```python
from build123d import *

# Parameters (mm, degrees)
SKETCH_1_W          = 25
SKETCH_1_H          = 2
EXTRUDE_1_DEPTH     = 20
SKETCH_1_3_W        = 25
SKETCH_1_3_H        = 10
SKETCH_1_3_R        = 1.5
EXTRUDE_2_DEPTH     = 2
SKETCH_2_R          = 1.5
CUT_EXTRUDE_1_DEPTH = 2


with BuildPart() as part:
    # Sketch 1 → Extrude 1 (new body)
    with BuildSketch(Plane(origin=(0, 0, 0), x_dir=(1, 0, 0), z_dir=(0, 1, 0))):
        with Locations((0, 4)):
            Rectangle(SKETCH_1_W, SKETCH_1_H)
    extrude(amount=EXTRUDE_1_DEPTH)

    # Sketch 1_3 → Extrude 2 (add)
    with BuildSketch(Plane(origin=(0, 0, 0), x_dir=(1, 0, 0), z_dir=(0, 1, 0))):
        Rectangle(SKETCH_1_3_W, SKETCH_1_3_H)
        with Locations(Location((-7.5, 0.997487313, 0), (0, 0, 270))):
            Circle(SKETCH_1_3_R, mode=Mode.SUBTRACT)
        with Locations(Location((7.5, 0.997487313, 0), (0, 0, 270))):
            Circle(SKETCH_1_3_R, mode=Mode.SUBTRACT)
    extrude(amount=EXTRUDE_2_DEPTH)

    # Sketch 2 → Cut-Extrude 1 (cut)
    with BuildSketch(Plane.XY.offset(-3)):
        with Locations((-7.5, 16.745611825)):
            Circle(SKETCH_2_R)
        with Locations((7.5, 16.745611825)):
            Circle(SKETCH_2_R)
    extrude(amount=-CUT_EXTRUDE_1_DEPTH, mode=Mode.SUBTRACT)


solid = part.part
```
CAD build for the part. Positions are in the model's coordinates, mm. A direction names the side the tool comes from. Coordinates: 2 decimals unless noted, no trailing zeros. Order: outer loops, then holes, each group sorted by start corner. A loop starts at its lowest first (then second) coordinate and runs counter-clockwise, first axis right, second up. Notation, with made-up numbers: (84.25, 16) - (111.25, 16) arc R32 cw to (111.25, 44) - close; hole circle Ø11 at (72.25, 8). An arc over 180 degrees is marked (long way). Use a Markdown table: item, result. Add a question column.
(1) Pull direction Z, two halves, no side cores. Call faces 1 (the face through (0, 0, 0)), 2 (the face through (0, 11, -3)), 3 (the face through (-9, 1, -1)): +Z half, -Z half, draft (parallel to the pull), parting line (faces both ways), or undercut.
(2) Flat gauge pins, fed straight in: pin 1 (3 mm diameter, centred on x = -8.5, y = 17, fed in from -Z); pin 2 (2.5 mm diameter, centred on x = -2, z = 0.5, fed in from +Y); pin 3 (1 mm diameter, centred on x = 0, y = 3.5, fed in from +Z). Where does each tip first touch, or does it go through?
(3) Saw through at A-A (x = 7.5). Give the cut face in (y, z), then the cut area to 3 significant figures.
(4) Saw through at C-C (z = 2.5). Give the cut face in (x, y), then the cut area to 3 significant figures.
(5) Which spindle directions (+Z, -Z, +X, -X, +Y, -Y) get a long thin tool onto all of the face, cutting with end or side? Do faces 4 (the face through (0, 2, 1)), 5 (the face through (-12.5, 7, -3.3)). Say none if no direction does.
(6) Drill centre lines: line 1 along Y through (x, z) = (7.5, -4.6); line 2 along X through (y, z) = (16, -3.25); line 3 along Z through (x, y) = (2, 14.25). Where is each one in solid material? Low to high. Write a range as [from, to].
(7) Saw through at B-B (z = -1.75). Give the cut face in (x, y).
(8) Saw through at D-D (x = -5.5). Give the cut face in (y, z), then the cut area to 3 significant figures.
Solved:
| question | item | result |
|---|---|---|
| 1 | face 1 | draft |
| 1 | face 2 | +Z half |
| 1 | face 3 | undercut |
| 2 | pin 1 | stops at z = -5 |
| 2 | pin 2 | stops at y = 2 |
| 2 | pin 3 | stops at z = -3 |
| 3 | outline | (0, -5) - (15.25, -5) - (15.25, -3) - (2, -3) - (2, -2.5) - (0, -2.5) - close; (0, 0.5) - (2, 0.5) - (2, 5) - (0, 5) - close; (18.25, -5) - (20, -5) - (20, -3) - (18.25, -3) - close |
| 3 | area | 44.0 mm² |
| 4 | outline | (-12.5, 0) - (12.5, 0) - (12.5, 2) - (-12.5, 2) - close |
| 4 | area | 50.0 mm² |
| 5 | face 4 | +Z, +X, -X, +Y |
| 5 | face 5 | +Z, -Z, -X, +Y, -Y |
| 6 | line 1 | y = [0, 15.25], [18.25, 20] |
| 6 | line 2 | x = [-12.5, -8.8], [-6.2, 6.2], [8.8, 12.5] |
| 6 | line 3 | z = [-5, -3] |
| 7 | outline | (-12.5, 0) - (-8.8, 0) - (-8.8, 2) - (-12.5, 2) - close; (-6.2, 0) - (6.2, 0) - (6.2, 2) - (-6.2, 2) - close; (8.8, 0) - (12.5, 0) - (12.5, 2) - (8.8, 2) - close |
| 8 | outline | (0, -5) - (20, -5) - (20, -3) - (2, -3) - (2, 5) - (0, 5) - close |
| 8 | area | 56.0 mm² |
